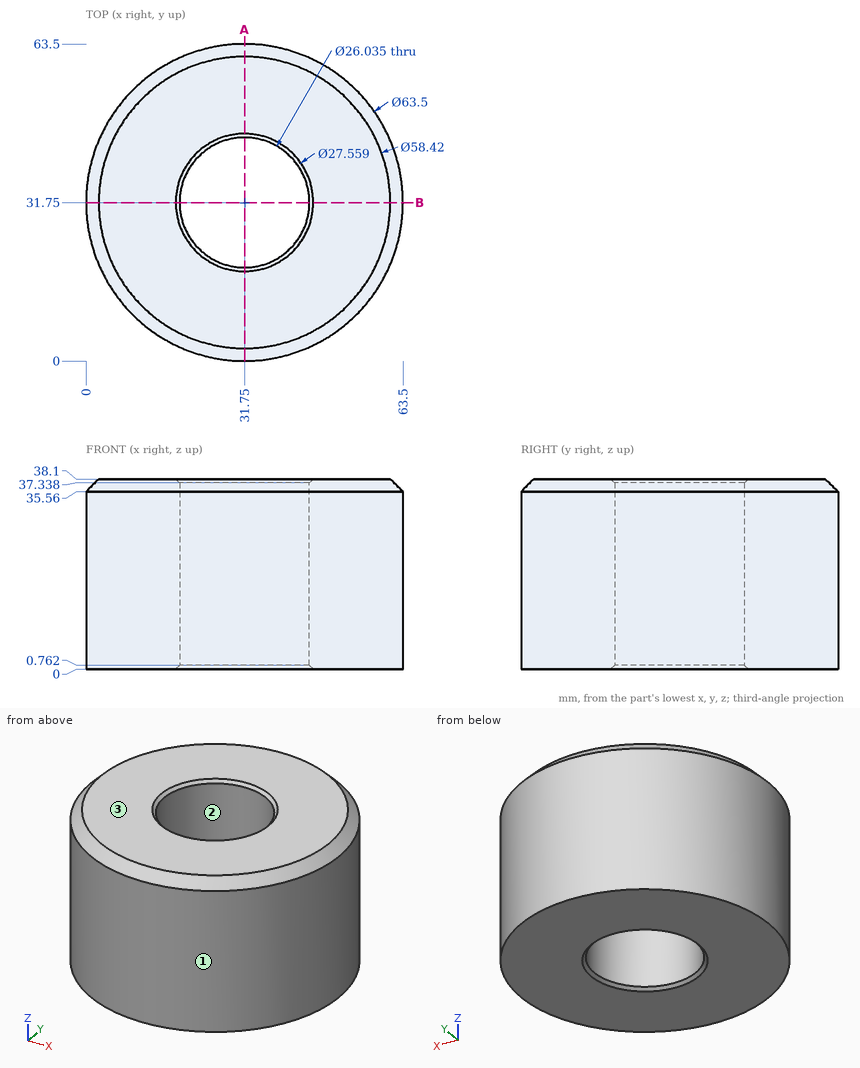
Drawing for the job (mm, zero at the part's lowest x, y, z). Coordinates: 2 decimals unless noted, no trailing zeros. Write each loop counter-clockwise with the first axis right and the second up, starting at its lowest first coordinate (ties: lowest second). Pieces come first, ordered by that corner, then holes. Notation, with made-up numbers: (60, -34.5) -> (77, -34.5) arc R24 cw to (77, -19.5) -> close; hole circle Ø9 at (-6.5, 50). An arc over 180 degrees is marked (long way). One line per item, written item: value. Start each with the question number.
1) Flat gauge pins, fed straight in: pin 1 Ø12 at (x, z) = (45, 8.5) entering from -Y; pin 2 Ø10 at (x, z) = (53.5, 27) entering from +Y; pin 3 Ø6 at (x, z) = (38.5, 18.5) entering from +Y. Where does each tip first touch, or does it go through?
2) Slice it at A-A on x = 31.75. Write the cut outline in (y, z), then the cut area to 3 significant figures.
3) Probe probe 1 along Y at (x, z) = (31.75, 23); probe 2 along X at (y, z) = (25.5, 3.5); probe 3 along X at (y, z) = (33, 23). List the from-to ranges inside material, lowest first.
4) Pull direction X, two halves, no side cores. Call the marked faces 1, 2 and 3: +X half, -X half, draft (parallel to the pull), parting line (faces both ways), or undercut.
Answers follow:
1. pin 1: y = 0.84
1. pin 2: y = 58.72
1. pin 3: y = 63.28
2. outline: (0, 0) -> (17.97, 0) -> (18.73, 0.76) -> (18.73, 37.34) -> (17.97, 38.1) -> (2.54, 38.1) -> (0, 35.56) -> close; (44.77, 0.76) -> (45.53, 0) -> (63.5, 0) -> (63.5, 35.56) -> (60.96, 38.1) -> (45.53, 38.1) -> (44.77, 37.34) -> close
2. area: 1,420 mm2
3. probe 1: 0 to 18.73, 44.77 to 63.5
3. probe 2: 0.62 to 20.33, 43.17 to 62.88
3. probe 3: 0.02 to 18.79, 44.71 to 63.48
4. face 1: parting line
4. face 2: undercut
4. face 3: draft
